from build123d import *

# Parameters (mm, degrees)
CROQUIS1_R              = 1.49817269
CROQUIS1_R_2            = 2.996164088
CROQUIS1_R_3            = 0.749999538
CROQUIS1_R_4            = 0.749999677
CROQUIS1_R_5            = 0.500000135
CROQUIS1_R_6            = 0.499999787
SALIENTE_EXTRUIR1_DEPTH = 4


with BuildPart() as part:
    # Croquis1 → Saliente-Extruir1 (new body)
    with BuildSketch(Plane(origin=(0, 0, 0), x_dir=(1, 0, 0), z_dir=(0, 1, 0))):
        with BuildLine():
            Line((-2.771145689, 3.732352208), (-1.295728101, 3.732352208))
            Line((-1.295728101, 3.732352208), (-1.295728101, 19.296313944))
            ThreePointArc((-1.295728101, 19.296313944), (1.809273381, 22.401315426), (4.914274862, 19.296313944))
            Line((4.914274862, 19.296313944), (4.914274862, -0.374323426))
            ThreePointArc((4.914274862, -0.374323426), (11.296230277, -12.207784547), (-0.100533102, -19.340381653))
            Line((-0.100533102, -19.340381653), (-0.473678479, -21.235402092))
            ThreePointArc((-0.473678479, -21.235402092), (-3.656560928, -22.956227452), (-4.742951437, -19.504889123))
            Line((-4.742951437, -19.504889123), (-3.638068078, -17.802867047))
            ThreePointArc((-3.638068078, -17.802867047), (-3.393654936, -16.784225076), (-3.844679826, -15.838738006))
            Line((-3.844679826, -15.838738006), (-4.320831306, -15.362586526))
            ThreePointArc((-4.320831306, -15.362586526), (-5.27515607, -14.910658594), (-6.299806788, -15.165738025))
            Line((-6.299806788, -15.165738025), (-7.976088157, -16.28110044))
            ThreePointArc((-7.976088157, -16.28110044), (-11.450003687, -15.233750996), (-9.768409722, -12.018588215))
            Line((-9.768409722, -12.018588215), (-7.77884303, -11.596670181))
            ThreePointArc((-7.77884303, -11.596670181), (-6.868732518, -11.039395013), (-6.512384859, -10.033475979))
            Line((-6.512384859, -10.033475979), (-6.512384859, -9.385437189))
            ThreePointArc((-6.512384859, -9.385437189), (-6.862343771, -8.397552686), (-7.756137447, -7.850268577))
            Line((-7.756137447, -7.850268577), (-9.756013297, -7.426164328))
            ThreePointArc((-9.756013297, -7.426164328), (-11.437933851, -4.204098724), (-7.955506206, -3.163300372))
            Line((-7.955506206, -3.163300372), (-6.292102369, -4.277795727))
            ThreePointArc((-6.292102369, -4.277795727), (-5.254751387, -4.534795839), (-4.293390141, -4.067965387))
            Line((-4.293390141, -4.067965387), (-3.797367558, -3.557739732))
            ThreePointArc((-3.797367558, -3.557739732), (-3.359699549, -2.605638888), (-3.61887602, -1.590317826))
            Line((-3.61887602, -1.590317826), (-4.728201004, 0.065299063))
            ThreePointArc((-4.728201004, 0.065299063), (-4.849446935, 2.48575952), (-2.771145689, 3.732352208))
        make_face()
        with Locations((1.806542391, 19.29086522)):
            Circle(CROQUIS1_R, mode=Mode.SUBTRACT)
        with Locations((1.80610831, -9.704394827)):
            Circle(CROQUIS1_R_2, mode=Mode.SUBTRACT)
        with Locations((0.059270172, -2.708668348)):
            Circle(CROQUIS1_R_3, mode=Mode.SUBTRACT)
        with Locations((3.559270137, -2.708669201)):
            Circle(CROQUIS1_R_4, mode=Mode.SUBTRACT)
        with Locations((0.059269976, -16.208667718)):
            Circle(CROQUIS1_R_5, mode=Mode.SUBTRACT)
        with Locations((3.559270485, -16.208667851)):
            Circle(CROQUIS1_R_6, mode=Mode.SUBTRACT)
    extrude(amount=SALIENTE_EXTRUIR1_DEPTH)


solid = part.part
Source: CAD feature listing. Evaluate the final solid. Frame: model axes, mm. A direction names the side the tool comes from. Coordinates: 2 decimals unless noted, no trailing zeros. Loops run counter-clockwise (first coordinate to the right, second up) from the corner with the lowest first, then second, coordinate; pieces in that order, holes last. Notation, with made-up numbers: (83.5, 13.25) - (127.5, 13.25) arc R18 cw to (127.5, 39.25) - close; hole circle Ø6 at (9.25, 17.25). An arc over 180 degrees is marked (long way). One line per item, written item: value. Start each with the question number.
1. Section D-D (x = 5.75). Return the cut outline in (y, z).
2. Ray query, L1, parallel to X at y = 1.05, z = 3; L2, parallel to X at y = 3.15, z = -7; L3, parallel to Z at x = -4.5, y = 3.4. Return the intervals inside material, ascending.
3. Section B-B (y = 2.1). State how many separate pieces and enclosed holes the cut face has, and give its area (3 significant figures).
4. Contact query for flat-ended pins moving along their axis: P1, Ø1.9, axis at x = 3.56, z = 2.71, coming from the +Y side; P2, Ø0.7, axis at y = 2.5, z = 9.5, coming from the -X side; P3, Ø0.9, axis at x = 0.06, z = 16.21, coming from the +Y side; P4, Ø1.5, axis at x = -6, y = 1, coming from the +Z side. Output: stop coordinate, or through.
5. Section A-A (x = -9). Return the cut outline in (y, z), and give its area (3 significant figures).
6. Set-up query: faces 1 (the flat face through (0, 0, 5)), 2 (the flat face through (-2, 2, -3.732)), 3 (the flat face through (-4.17, 1.97, 0.77)), 4 (the cylindrical face through (-3.36, 1.97, 2.62)), 5 (the flat face through (0, 4, 5)). Return all of +Z, -Z, +X, -X, +Y, -Y with unobstructed straight access to the full face (end or side cutting, diameter ignored); none if empty.
7. Section C-C (z = -8). Return the cut outline in (x, y), and give its area (3 significant figures).
8. Mould query, pull axis Z, two halves, no side actions, for faces 6 (the flat face through (-1.296, 2, -11)), 7 (the flat face through (-7.14, 1.97, 3.71)), 8 (the cylindrical face through (-5.26, 1.972, 14.912)), 9 (the flat face through (-4.2, 1.97, 18.67)). Classes: pulls with the +Z half, pulls with the -Z half, needs draft (parallel to the pull), parting line crosses it, or undercut.
Verdict:
1. outline: (0, 0.7) - (4, 0.7) - (4, 18.69) - (0, 18.69) - close
2. L1: x = -10.29 to -8.24, -3.45 to -0.63, 0.75 to 2.87, 4.25 to 8.99
2. L2: x = -1.3 to 4.91
2. L3: z = -2.98 to 0.28, 4.25 to 15.21, 19.13 to 22.37
3. separate pieces: 1
3. enclosed holes: 6
3. area: 456 mm2
4. P1: stops at y = 4
4. P2: stops at x = -6.53
4. P3: passes through
4. P4: stops at z = 15.47
5. outline: (0, 2.78) - (4, 2.78) - (4, 7.59) - (0, 7.59) - close; (0, 11.86) - (4, 11.86) - (4, 16.66) - (0, 16.66) - close
5. area: 38.4 mm2
6. face 1: +Z, -Z, +X, -X, -Y
6. face 2: -Z, -X, +Y, -Y
6. face 3: -X, +Y, -Y
6. face 4: +Y, -Y
6. face 5: +Z, -Z, +X, -X, +Y
7. outline: (-1.3, 0) - (4.91, 0) - (4.91, 4) - (-1.3, 4) - close
7. area: 24.8 mm2
8. face 6: needs draft
8. face 7: pulls with the -Z half
8. face 8: undercut
8. face 9: undercut
